Can you work these out from the model? Positions are in its coordinate system, mm. Give positions to 0.01 mm unless a question says otherwise; leave off trailing zeros. Write each loop counter-clockwise with the first axis right and the second up, starting at its lowest first coordinate (ties: lowest second). Pieces come first, ordered by that corner, then holes.
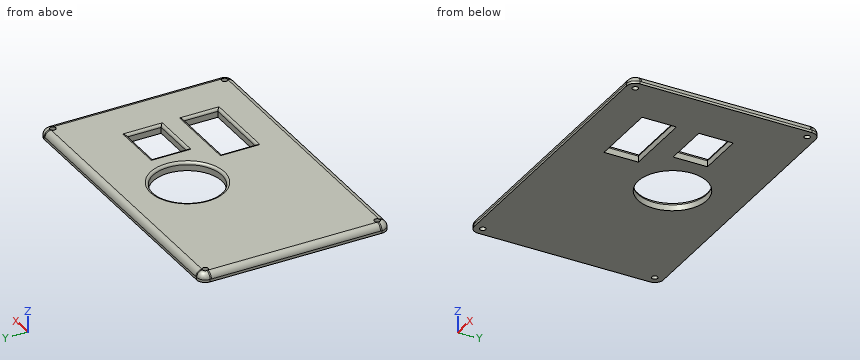
Autodesk Fusion 360 part; units mm, degrees
sketch "Sketch1" plane through (0, 0, 0) normal (0, 0, 1) x (1, 0, 0) in component "FloppySquare Top (1)"
  line L0 (0, 0) -> (170, 0)
  line L1 (170, 0) -> (170, 110)
  line L2 (170, 110) -> (0, 110)
  line L3 (0, 110) -> (0, 0)
  circle A0 centre (5, 105) radius 1.7
  circle A1 centre (5, 5) radius 1.7
  circle A2 centre (165, 105) radius 1.7
  circle A3 centre (165, 5) radius 1.7
  line L4 (141.5, 75) -> (114.5, 75)
  line L5 (114.5, 75) -> (114.5, 55)
  line L6 (114.5, 55) -> (141.5, 55)
  line L7 (141.5, 55) -> (141.5, 75)
  circle A4 centre (85, 71) radius 20
  line L8 (141.5, 22) -> (101.5, 22)
  line L9 (101.5, 22) -> (101.5, 42)
  line L10 (101.5, 42) -> (141.5, 42)
  line L11 (141.5, 42) -> (141.5, 22)
  dimension "d1" = 170
  dimension "d2" = 110
  dimension "d3" = 3.4
  dimension "d4" = 3.4
  dimension "d5" = 3.4
  dimension "d6" = 3.4
  dimension "d7" = 5
  dimension "d8" = 5
  dimension "d9" = 5
  dimension "d10" = 5
  dimension "d11" = 5
  dimension "d12" = 5
  dimension "d13" = 5
  dimension "d14" = 5
  dimension "d15" = 27
  dimension "d16" = 20
  dimension "d17" = 28.5
  dimension "d18" = 35
  dimension "d19" = 40
  dimension "d20" = 85
  dimension "d21" = 39
  dimension "d22" = 40
  dimension "d23" = 20
  dimension "d24" = 22
  dimension "d25" = 28.5
extrude "Extrude1" add sketch "Sketch1" along normal blind 5 in component "FloppySquare Top (1)"
fillet "Fillet1" radius 5 4 edges at (0, 110, 2.5) (0, 0, 2.5) (170, 0, 2.5) (170, 110, 2.5) in component "FloppySquare Top (1)"
fillet "Fillet2" radius 3.5 8 edges at (1.4645, 108.5355, 5) (0, 55, 5) (1.4645, 1.4645, 5) (85, 0, 5) (168.5355, 1.4645, 5) (170, 55, 5) (168.5355, 108.5355, 5) (85, 110, 5) in component "FloppySquare Top (1)"
fillet "Fillet3" radius 1.5 9 edges at (141.5, 65, 5) (128, 55, 5) (114.5, 65, 5) (128, 75, 5) (121.5, 42, 5) (141.5, 32, 5) (101.5, 32, 5) (121.5, 22, 5) (66.3535, 78.2323, 5) in component "FloppySquare Top (1)"
component "FloppySquare Top (1)" placed x (1, 0, 0) y (0, 1, 0) z (0, 0, 1) at (0, 0, 0)
(1) Imagine slicing it at B-B, the plane y = 34.5. Write out the boundary of the cut face in (x, z), plus the area to 3 significant figures.
Returned:
outline: (0, 0) - (101.5, 0) - (101.5, 3.5) arc R1.5 ccw to (100, 5) - (3.5, 5) arc R3.5 ccw to (0, 1.5) - close; (141.5, 0) - (170, 0) - (170, 1.5) arc R3.5 ccw to (166.5, 5) - (143, 5) arc R1.5 ccw to (141.5, 3.5) - close
area: 644 mm2
(2) Imagine slicing it at A-A, the plane y = 71. Write out the boundary of the cut face in (x, z).
Returned:
outline: (0, 0) - (65, 0) - (65, 3.5) arc R1.5 ccw to (63.5, 5) - (3.5, 5) arc R3.5 ccw to (0, 1.5) - close; (105, 0) - (114.5, 0) - (114.5, 3.5) arc R1.5 ccw to (113, 5) - (106.5, 5) arc R1.5 ccw to (105, 3.5) - close; (141.5, 0) - (170, 0) - (170, 1.5) arc R3.5 ccw to (166.5, 5) - (143, 5) arc R1.5 ccw to (141.5, 3.5) - close
(3) Imagine slicing it at C-C, the plane z = 2.35. Give the number of separate pieces and of enclosed holes in the cut face, plus the area to 3 significant figures.
Returned:
separate pieces: 1
enclosed holes: 7
area: 16,000 mm2
(4) Will these pins go through, and if not, where does the flat tip stop? P1, Ø5.5, axis at x = 5, y = 105, coming from the +Z side; P2, Ø1.5, axis at y = 74, z = 2.5, coming from the +X side; P3, Ø2, axis at x = 133, z = 3.5, coming from the +Y side; P4, Ø2.5, axis at x = 165, y = 5, coming from the +Z side.
Returned:
P1: stops at z = 5
P2: stops at x = 169.99
P3: stops at y = 109.85
P4: passes through
(5) If I drill on L1, parallel to X at y = 5, z = 1.95; L2, parallel to Y at x = 165, z = 1; L3, parallel to X at y = 71.5, z = 3.4, over which ranges is the centre line in solid material (lowest first)?
Returned:
L1: x = 0.03 to 3.3, 6.7 to 163.3, 166.7 to 169.97
L2: y = 0 to 3.3, 6.7 to 103.3, 106.7 to 110
L3: x = 0.56 to 65.01, 104.99 to 114.5, 141.5 to 169.44
